Check sheet for the modelled part. Datum: model origin and axes. Units: mm. Face numbers are marked on the shaded views. A direction names the side the tool comes from. Round coordinates to 2 decimals unless told otherwise and drop trailing zeros. Loops run counter-clockwise (first coordinate to the right, second up) from the corner with the lowest first, then second, coordinate; pieces in that order, holes last. Notation, with made-up numbers: M 70,39 L 111,39 A10 cw 111,47 Z; hole C 5.25,82.25 d7. An arc over 180 degrees is marked long. Write item = value, one per line. Start each with the question number.
(1) Mould release check, pull along X, two halves, no side actions. Record for the marked faces 4, 5 and 6: pulls with the +X half, pulls with the -X half, needs draft (parallel to the pull), parting line crosses it, or undercut.
(2) Set-up check for the marked faces 1, 2 and 3: record each of +Z, -Z, +X, -X, +Y, -Y from which the full face is reachable in a straight line by a thin tool's end or side.
(3) Cross-section at C-C on x = -2. Record the boundary of the cut face in (y, z) (3 decimals).
(4) Cross-section at D-D on x = 25. Record the boundary of the cut face in (y, z) (3 decimals).
(5) Cross-section at B-B on z = -29.5. Record the boundary of the cut face in (x, y), plus the area to 3 significant figures.
(6) Scan lines: L1, parallel to Z at x = 30.5, y = -71 (3 decimals); L2, parallel to Z at x = 41, y = -17.5; L3, parallel to Z at x = -5, y = -32.5 (3 decimals). Record each from-to range of solid material in increasing order. Write a range as from..to.
(7) Go/stop test with flat-tipped pins: P1, Ø7.5, axis at x = 9.5, y = -7, coming from the +Z side; P2, Ø21.5, axis at x = 17, z = 2.5, coming from the -Y side. Record where each tip stops, or that it passes through.
(8) Cross-section at A-A on y = -68.5. Record the boundary of the cut face in (x, z) (3 decimals).
from build123d import *

# Parameters (mm, degrees)
F0_R     = 12.7
F1_DEPTH = 25.4
F0_W     = 38.1
F0_H     = 19.960821
F0_W_2   = 76.2
F0_H_2   = 10.794998
F2_DEPTH = 76.2


with BuildPart() as f1:
    # F0 (on Front) → F1 (new body)
    with BuildSketch(Plane.XZ):
        Polygon((60.409845, 30.839179), (22.309845, 30.839179), (22.309845, 0), (-15.790155, 0), (-15.790155, -40.005002), (60.409845, -40.005002), (60.409845, 0), align=None)
        with Locations((8.306528, -26.447218)):
            Circle(F0_R, mode=Mode.SUBTRACT)
        with Locations((41.532636, 0)):
            Circle(F0_R, mode=Mode.SUBTRACT)
    extrude(amount=F1_DEPTH)

    # F0 (on Front) → F2 (join)
    with BuildSketch(Plane.XZ):
        with Locations((41.359845, 40.819589)):
            Rectangle(F0_W, F0_H)
        with Locations((22.309845, -45.402501)):
            Rectangle(F0_W_2, F0_H_2)
    extrude(amount=F2_DEPTH)


solid = f1.part
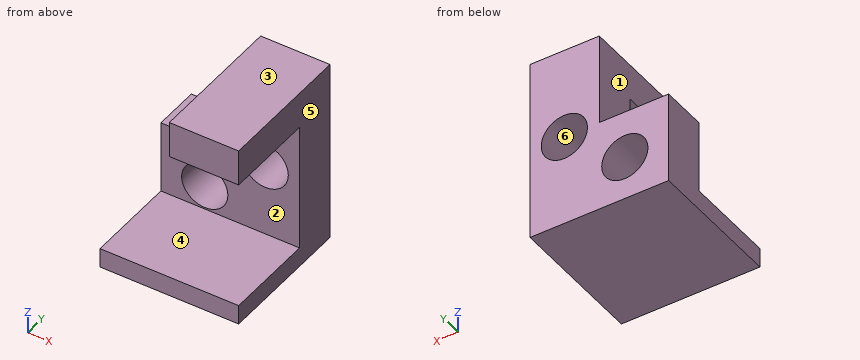
Result:
q1.face_4 = needs draft
q1.face_5 = pulls with the +X half
q1.face_6 = undercut
q2.face_1 = +Z, -X, +Y, -Y
q2.face_2 = +X, -X, -Y
q2.face_3 = +Z, +X, -X, +Y, -Y
q3.outline = M -76.2,-50.8 L 0,-50.8 L 0,-33.868 L -25.4,-33.868 L -25.4,-40.005 L -76.2,-40.005 Z; M -25.4,-19.027 L 0,-19.027 L 0,0 L -25.4,0 Z
q4.outline = M -76.2,-50.8 L 0,-50.8 L 0,50.8 L -76.2,50.8 L -76.2,30.839 L -25.4,30.839 L -25.4,-40.005 L -76.2,-40.005 Z
q5.outline = M -15.79,-25.4 L -4.02,-25.4 L -4.02,0 L -15.79,0 Z; M 20.63,-25.4 L 60.41,-25.4 L 60.41,0 L 20.63,0 Z
q5.area = 1,310 mm^2
q6.L1 = -50.8..-40.005, 30.839..50.8
q6.L2 = -50.8..-12.69, 12.69..50.8
q6.L3 = -50.8..-40.005
q7.P1 = 0
q7.P2 = -25.4
q8.outline = M -15.79,-50.8 L 60.41,-50.8 L 60.41,-40.005 L -15.79,-40.005 Z; M 22.31,30.839 L 60.41,30.839 L 60.41,50.8 L 22.31,50.8 Z
